```python
from build123d import *

# Parameters (mm, degrees)
F0_W     = 56.642
F0_H     = 31.75
F1_DEPTH = 31.75
F2_R     = 10.16
F3_DEPTH = 13.4874
F4_R     = 7.9375
F5_DEPTH = 16.002
F5_TAPER = 3
F7_D     = 5.4102
F7_DEPTH = 27.94
F7_TIP   = 1.6253880605


with BuildPart() as f1:
    # F0 (on Top) → F1 (new body)
    with BuildSketch(Plane.XY):
        with Locations((-28.321, -15.875)):
            Rectangle(F0_W, F0_H)
    extrude(amount=-F1_DEPTH)

    # F2 (on face) → F3 (join)
    with BuildSketch(Plane(origin=(-56.642, 0, 0), x_dir=(0, -1, 0), z_dir=(-1, 0, 0))):
        with Locations((15.875, -15.875)):
            Circle(F2_R)
    extrude(amount=F3_DEPTH)

    # F4 (on face) → F5 (join)
    with BuildSketch(Plane(origin=(-70.1294, 0, 0), x_dir=(0, -1, 0), z_dir=(-1, 0, 0))):
        with Locations((15.875, -15.875)):
            Circle(F4_R)
    extrude(amount=F5_DEPTH, taper=F5_TAPER)

    # F7
    with Locations(Plane.XY):
        with Locations((-15.0622, -15.875), (-40.4622, -15.875)):
            Hole(F7_D / 2, depth=F7_DEPTH)
            with Locations((0, 0, -(F7_DEPTH + F7_TIP / 2))):  # 118° drill point
                Cone(0, F7_D / 2, F7_TIP, mode=Mode.SUBTRACT)


solid = f1.part
```
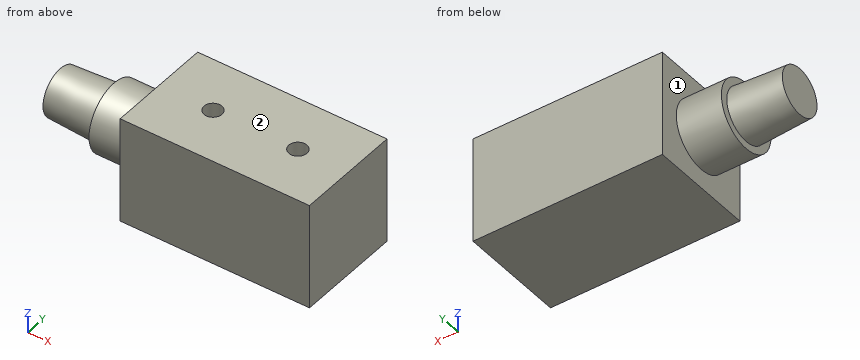
Design review of the part built by this model. Coordinates are the model's own, in mm. Face numbers are marked on the shaded views. A direction names the side the tool comes from. Coordinates: 2 decimals unless noted, no trailing zeros. Order: outer loops, then holes, each group sorted by start corner. A loop starts at its lowest first (then second) coordinate and runs counter-clockwise, first axis right, second up.
1) For the marked faces 1 and 2, list the 3-axis set-ups (+Z, -Z, +X, -X, +Y, -Y) from which the entire face can be reached by the end or side of a thin tool; tool diameter is ignored.
2) Wall thickness on line 1 along X through (y, z) = (-16, -1.5); line 2 along X through (y, z) = (-13.5, -15); line 3 along X through (y, z) = (-25, -24): over which ranges is each line inside the solid? List them lowest first.
3) Take a section at B-B, the plane y = -4.5. Give the boundary of the cut face in (x, z).
4) Take a section at D-D, the plane z = -17. State how many separate pieces and enclosed holes the cut face has, and give its area (3 significant figures).
5) Take a section at A-A, the plane z = -3.5. Give the boundary of the cut face in (x, y) (3 decimals), and give its area (3 significant figures).
6) Take a section at C-C, the plane x = -78. Give the boundary of the cut face in (y, z) (3 decimals), and give its area (3 significant figures).
7) Clearance check with flat-ended pins moving along their axes: pin 1 (10 mm diameter, centred on y = -25.5, z = -4.5, fed in from -X); pin 2 (5 mm diameter, centred on x = -60, y = -19.5, fed in from -Z). State where each tip first meets the part, or that it passes through.
Returned:
1. face 1: -X
1. face 2: +Z, +X, -X, +Y, -Y
2. line 1: x = -56.64 to -43.16, -37.76 to -17.76, -12.36 to 0
2. line 2: x = -86.13 to -41.76, -39.17 to -16.36, -13.77 to 0
2. line 3: x = -56.64 to 0
3. outline: (-56.64, -31.75) - (0, -31.75) - (0, 0) - (-56.64, 0) - close
4. separate pieces: 1
4. enclosed holes: 2
4. area: 2,260 mm2
5. outline: (-56.642, -31.75) - (0, -31.75) - (0, 0) - (-56.642, 0) - close; hole circle Ø5.41 at (-40.462, -15.875); hole circle Ø5.41 at (-15.062, -15.875)
5. area: 1,750 mm2
6. outline: circle Ø15.05 at (-15.875, -15.875)
6. area: 178 mm2
7. pin 1: stops at x = -70.13
7. pin 2: stops at z = -25.97
